For this review, use the dimensioned drawing (mm, ordinates from the lowest corner) and the shaded views. Coordinates: 2 decimals unless noted, no trailing zeros. Write each loop counter-clockwise with the first axis right and the second up, starting at its lowest first coordinate (ties: lowest second). Pieces come first, ordered by that corner, then holes. Notation, with made-up numbers: (10, 36) -> (42, 36) arc R30 ccw to (42, 72) -> close; hole circle Ø4 at (43.25, -4.75). An arc over 180 degrees is marked (long way). Put each result on its own line as item: value. Start each with the question number.
Item 1: Consider section D-D on z = 8.5. Give the boundary of the cut face in (x, y), and give its area (3 significant figures).
Item 2: To check wall thickness, follow L1, parallel to Y at x = 2.8, z = 42; L2, parallel to Z at x = 2.45, y = 42.5; L3, parallel to Z at x = 1.3, y = 39. State the ranges of each line that lie inside material, in increasing order.
Item 3: Consider section A-A on x = 1.45. Give the boundary of the cut face in (y, z).
Item 4: Consider section C-C on y = 48.5. Give the boundary of the cut face in (x, z).
Item 5: Insertion check: P1, Ø1.5, axis at y = 21, z = 13, coming from the -X side; P2, Ø1.5, axis at x = 2, y = 42.5, coming from the -Z side; P3, Ø1.5, axis at x = 2, y = 38, coming from the +Z side. Each pin has a flat end and moves straight along its axis. Give the tip position at first contact, or say it passes through.
Item 6: Consider section B-B on z = 26. Give the boundary of the cut face in (x, y).
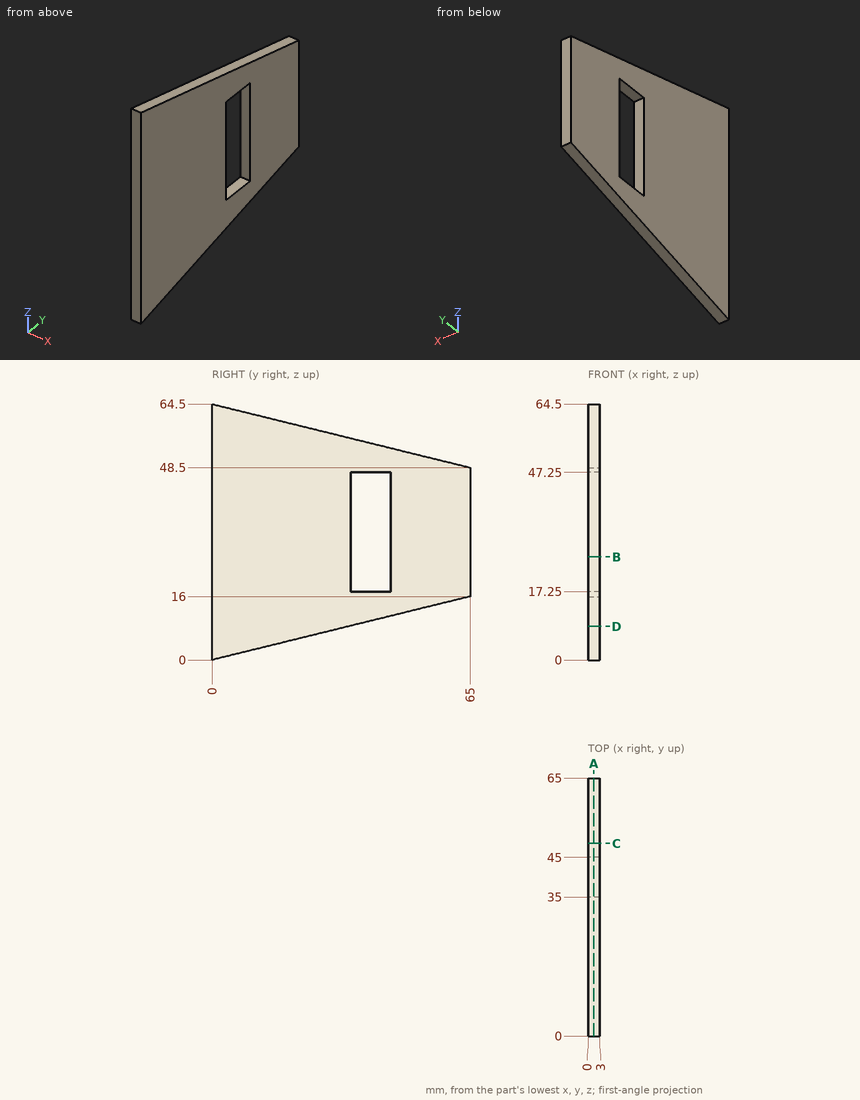
Return value:
1. outline: (0, 0) -> (3, 0) -> (3, 34.53) -> (0, 34.53) -> close
1. area: 104 mm^2
2. L1: 0 to 35, 45 to 65
2. L2: 10.46 to 17.25, 47.25 to 54.04
2. L3: 9.6 to 17.25, 47.25 to 54.9
3. outline: (0, 0) -> (65, 16) -> (65, 48.5) -> (0, 64.5) -> close; hole (35, 17.25) -> (45, 17.25) -> (45, 47.25) -> (35, 47.25) -> close
4. outline: (0, 11.94) -> (3, 11.94) -> (3, 52.56) -> (0, 52.56) -> close
5. P1: x = 0
5. P2: z = 10.28
5. P3: z = 55.33
6. outline: (0, 0) -> (3, 0) -> (3, 35) -> (0, 35) -> close; (0, 45) -> (3, 45) -> (3, 65) -> (0, 65) -> close
